Drawing for the job (mm, zero at the part's lowest x, y, z). A direction names the side the tool comes from. Give positions to 0.01 mm unless a question says otherwise; leave off trailing zeros. Order: outer loops, then holes, each group sorted by start corner. A loop starts at its lowest first (then second) coordinate and runs counter-clockwise, first axis right, second up. Notation, with made-up numbers: (82, 72.5) - (135, 72.5) arc R31 ccw to (135, 107.5) - close; hole circle Ø11 at (79, 56.5). An arc over 180 degrees is marked (long way). Use a Markdown table: item, result. Add a question column.
(1) Flat gauge pins, fed straight in: pin 1 (5 mm diameter, centred on x = 2.5, z = 13.5, fed in from -Y); pin 2 (8 mm diameter, centred on x = 13, z = 8.5, fed in from +Y); pin 3 (1 mm diameter, centred on x = 15, z = 6.5, fed in from -Y); pin 4 (3 mm diameter, centred on x = 7, y = 15, fed in from -Z). Where does each tip first touch, or does it go through?
(2) Which spindle directions (+Z, -Z, +X, -X, +Y, -Y) get a long thin tool onto all of the face, cutting with end or side? Do the marked faces 1 and 2. Say none if no direction does.
(3) Wall check: line 1 (Z direction, x = 5, y = 13.5); line 2 (Z direction, x = 4.5, y = 8.75); line 3 (Y direction, x = 8.25, z = 8). Give the ranges that are in metal, low to high.
(4) Slice it at A-A (x = 8.5). Write the cut outline in (y, z).
(5) Slice it at C-C (z = 3.5). Write the cut outline in (x, y).
(6) Slice it at D-D (x = 13). Write the cut outline in (y, z), then the cut area to 3 significant figures.
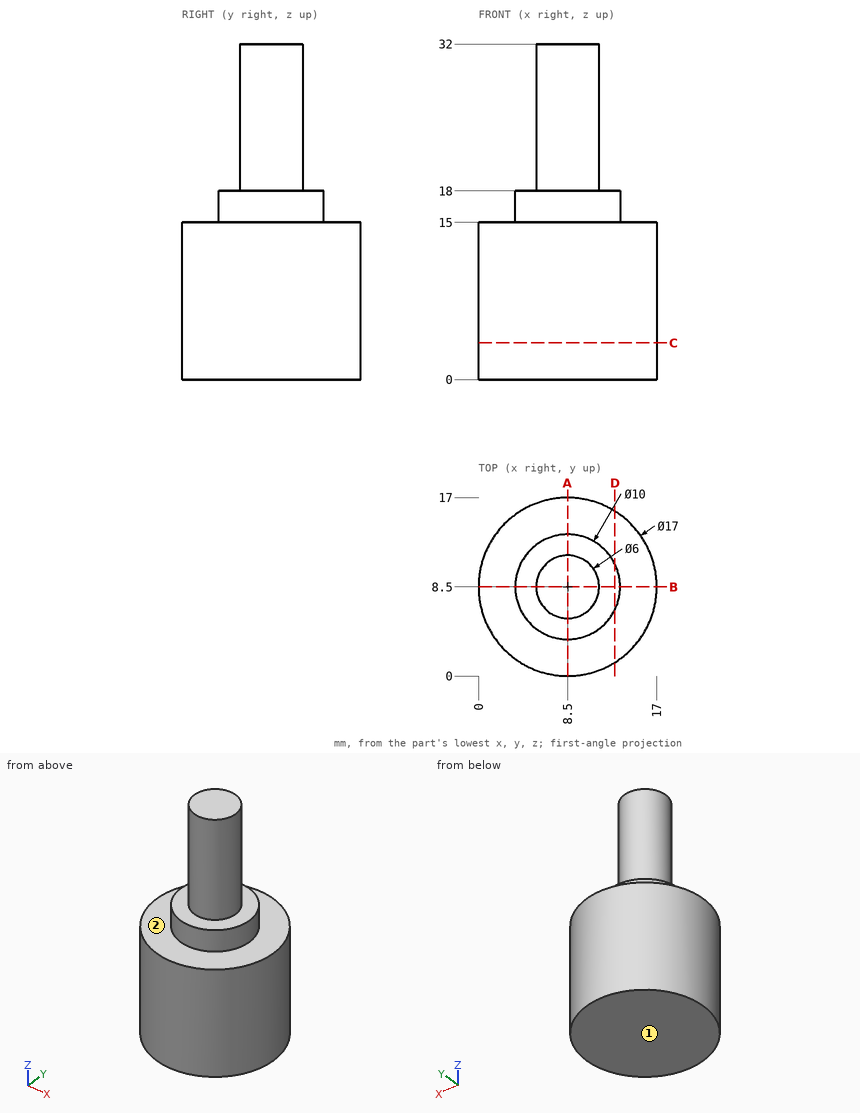
Solution:
| question | item | result |
|---|---|---|
| 1 | pin 1 | y = 0.75 |
| 1 | pin 2 | y = 16.99 |
| 1 | pin 3 | y = 2.48 |
| 1 | pin 4 | z = 0 |
| 2 | face 1 | -Z, +X, -X, +Y, -Y |
| 2 | face 2 | +Z |
| 3 | line 1 | 0 to 15 |
| 3 | line 2 | 0 to 18 |
| 3 | line 3 | 0 to 17 |
| 4 | outline | (0, 0) - (17, 0) - (17, 15) - (13.5, 15) - (13.5, 18) - (11.5, 18) - (11.5, 32) - (5.5, 32) - (5.5, 18) - (3.5, 18) - (3.5, 15) - (0, 15) - close |
| 5 | outline | circle Ø17 at (8.5, 8.5) |
| 6 | outline | (1.29, 0) - (15.71, 0) - (15.71, 15) - (10.68, 15) - (10.68, 18) - (6.32, 18) - (6.32, 15) - (1.29, 15) - close |
| 6 | area | 229 mm2 |
